Can you work these out from the model? Positions are in its coordinate system, mm. A direction names the side the tool comes from. Coordinates: 2 decimals unless noted, no trailing zeros. Loops run counter-clockwise (first coordinate to the right, second up) from the corner with the lowest first, then second, coordinate; pieces in that order, holes last. Notation, with made-up numbers: (-37, -17.75) - (-2, -17.75) arc R17 cw to (-2, -7.75) - close; hole circle Ø9 at (-40, 40.25). An arc over 180 degrees is marked (long way). Put each result on its own line as item: value. Start each with the question number.
from build123d import *

# Parameters (mm, degrees)
SKETCH1_W               = 8
SKETCH1_H               = 8
BOSS_EXTRUDE1_DEPTH     = 3
CUT_EXTRUDE1_DEPTH      = 12.704699911
CUT_EXTRUDE1_DEPTH_BACK = 12.704699911
CUT_EXTRUDE2_DEPTH      = 11
SKETCH4_R               = 1.75
CUT_EXTRUDE3_DEPTH      = 0.4
SKETCH5_W               = 8
SKETCH5_H               = 1
BOSS_EXTRUDE2_DEPTH     = 2
FILLET1_R               = 4
CUT_EXTRUDE4_DEPTH      = 0.4
CUT_EXTRUDE5_DEPTH      = 0.5


with BuildPart() as part:
    # Sketch1 → Boss-Extrude1 (new body)
    with BuildSketch(Plane(origin=(0, 0, 0), x_dir=(1, 0, 0), z_dir=(0, 1, 0))):
        with Locations((4, 4)):
            Rectangle(SKETCH1_W, SKETCH1_H)
    extrude(amount=BOSS_EXTRUDE1_DEPTH)

    # Sketch2 → Cut-Extrude1 (cut, two sides: drawn at the far end of the back side and taken through both)
    with BuildSketch(Plane.XY.offset(-CUT_EXTRUDE1_DEPTH_BACK)):
        Polygon((0, 0), (0.6, 3), (0, 3), align=None)
        Polygon((8, 0), (7.4, 3), (8, 3), align=None)
    extrude(amount=CUT_EXTRUDE1_DEPTH + CUT_EXTRUDE1_DEPTH_BACK, mode=Mode.SUBTRACT)

    # Sketch3 → Cut-Extrude2 (cut)
    with BuildSketch(Plane(origin=(0, 0, 0), x_dir=(0, 0, -1), z_dir=(1, 0, 0))):
        Polygon((0, 0), (0.6, 3), (0, 3), align=None)
        Polygon((8, 3), (7.4, 3), (8, 0), align=None)
    extrude(amount=CUT_EXTRUDE2_DEPTH, mode=Mode.SUBTRACT)

    # Sketch4 → Cut-Extrude3 (cut)
    with BuildSketch(Plane.XZ):
        with Locations(Location((4, -3.75, 0), (0, 0, 270))):
            Circle(SKETCH4_R)
    extrude(amount=-CUT_EXTRUDE3_DEPTH, mode=Mode.SUBTRACT)

    # Sketch5 → Boss-Extrude2 (add)
    with BuildSketch(Plane.XZ):
        with Locations((4, -7.5)):
            Rectangle(SKETCH5_W, SKETCH5_H)
    extrude(amount=BOSS_EXTRUDE2_DEPTH)

    # Fillet1
    # the kernel refuses this fillet: 4 mm, written as the material it takes off along each edge
    with BuildSketch(Plane(origin=(8, -2, -16.660254038), x_dir=(0, 1, 0), z_dir=(0, 0, 1)), Plane(origin=(0, -2, 1.660254038), x_dir=(0, 1, 0), z_dir=(0, 0, -1))) as fillet1_piece_1:
        with BuildLine():
            CenterArc((4, 3.464101615), FILLET1_R, 180, 60)
            Line((0, 3.464101615), (-0.08, 3.464101615))
            Line((-0.08, 3.464101615), (-0.08, 0))
            Line((-0.08, 0), (0, -0.08))
            ThreePointArc((0, -0.08), (1, -0.08), (1.96, -0.069282032))
            Line((1.96, -0.069282032), (2, 0))
        make_face()
    extrude(amount=18.320508076, mode=Mode.SUBTRACT)

    # Sketch6 → Cut-Extrude4 (cut)
    with BuildSketch(Plane(origin=(0, 3, 0), x_dir=(1, 0, 0), z_dir=(0, 1, 0))):
        with BuildLine():
            Line((2.312898911, 2.041410717), (2.312898911, 6.041410717))
            Line((2.312898911, 6.041410717), (3.991584808, 6.041410717))
            add(Edge.make_bspline(
                [(3.991584808, 6.041410717), (4.042601732, 6.041096301), (4.140920681, 6.040490364), (4.283109063, 6.036071747), (4.414238667, 6.026814487), (4.534891188, 6.016330564), (4.644487122, 6.001077132), (4.74345979, 5.982803671), (4.831642566, 5.961627249), (4.910322089, 5.936265049), (4.982061831, 5.90723713), (5.04889092, 5.87268574), (5.111544162, 5.83220454), (5.170983849, 5.787188805), (5.227461685, 5.737569368), (5.279429347, 5.682033053), (5.32779225, 5.621406813), (5.372511371, 5.556195062), (5.411906117, 5.48668575), (5.447902572, 5.415111184), (5.477205044, 5.340709703), (5.50140862, 5.263831792), (5.52074281, 5.184644366), (5.534162371, 5.102946099), (5.542540058, 5.018884869), (5.543287935, 4.962103945), (5.543668142, 4.93323764)],
                knots=[0, 0, 0, 0, 1.675828044, 3.229627355, 4.67171229, 5.993455049, 7.206927059, 8.304770529, 9.29850117, 10.183580433, 11.017754134, 11.837875825, 12.650738409, 13.464925643, 14.285328857, 15.117007378, 15.959673368, 16.830859064, 17.711229498, 18.58228265, 19.460420693, 20.334473227, 21.228207035, 22.135446768, 23.052097822, 24, 24, 24, 24], degree=3))
            add(Edge.make_bspline(
                [(5.543668142, 4.93323764), (5.542962916, 4.896874176), (5.541584712, 4.825809944), (5.528901745, 4.721651895), (5.5100643, 4.622136315), (5.483211668, 4.527125334), (5.446289845, 4.437736414), (5.403428122, 4.352717347), (5.352308317, 4.272356517), (5.293277733, 4.19745058), (5.226389218, 4.127933229), (5.151349641, 4.065235076), (5.06869476, 4.009111084), (4.977924564, 3.959884897), (4.879671091, 3.917801842), (4.77350828, 3.882394441), (4.659916733, 3.853576761), (4.580902516, 3.840017181), (4.540463013, 3.833077384)],
                knots=[0, 0, 0, 0, 1.05911256, 2.069797862, 3.05271628, 4.008392045, 4.940519534, 5.866323021, 6.779546087, 7.71056835, 8.640711998, 9.585328432, 10.554502533, 11.547017206, 12.589327225, 13.664782803, 14.804835066, 16, 16, 16, 16], degree=3))
            add(Edge.make_bspline(
                [(4.540463013, 3.833077384), (4.579572554, 3.807174767), (4.656115253, 3.756479818), (4.762017587, 3.672984601), (4.857092756, 3.585349912), (4.929078878, 3.507419696), (4.984392794, 3.438888442), (5.028929947, 3.378950347), (5.076970406, 3.309970293), (5.128042999, 3.231910907), (5.183657562, 3.145462828), (5.241745689, 3.049302835), (5.303522957, 2.944368887), (5.345058377, 2.871067212), (5.366584808, 2.833077384)],
                knots=[0, 0, 0, 0, 1.285445069, 2.515791127, 3.691898215, 4.826622834, 5.420063933, 6.105349801, 6.873086501, 7.723915395, 8.66222816, 9.690593598, 10.803111229, 12, 12, 12, 12], degree=3))
            Line((5.366584808, 2.833077384), (5.851360449, 2.041410717))
            Line((5.851360449, 2.041410717), (4.952321988, 2.041410717))
            Line((4.952321988, 2.041410717), (4.383411731, 2.949263281))
            add(Edge.make_bspline(
                [(4.383411731, 2.949263281), (4.357283981, 2.985622121), (4.307400733, 3.055038622), (4.235391184, 3.153681722), (4.169508837, 3.241491798), (4.111507042, 3.319740728), (4.058450932, 3.386209972), (4.011951502, 3.442057857), (3.972955886, 3.488482798), (3.928832249, 3.534515131), (3.877499082, 3.581823547), (3.813952721, 3.627691749), (3.748696505, 3.664257396), (3.678779681, 3.692157844), (3.597922987, 3.71161189), (3.500720436, 3.724006591), (3.384115753, 3.733151261), (3.299833928, 3.733519777), (3.254405321, 3.73371841)],
                knots=[0, 0, 0, 0, 1.465447777, 2.797841088, 3.997266218, 5.05856206, 5.985598736, 6.780315439, 7.437430484, 7.969193402, 8.866571936, 9.718200644, 10.52825214, 11.309096006, 12.174169268, 13.242355782, 14.513606761, 16, 16, 16, 16], degree=3))
            Line((3.254405321, 3.73371841), (3.08212968, 3.73371841))
            Line((3.08212968, 3.73371841), (3.08212968, 2.041410717))
            Line((3.08212968, 2.041410717), (2.312898911, 2.041410717))
        make_face()
        with BuildLine():
            Line((3.08212968, 4.400385076), (3.701520706, 4.400385076))
            add(Edge.make_bspline(
                [(3.701520706, 4.400385076), (3.749332843, 4.400487541), (3.840423044, 4.400682752), (3.969955122, 4.403510317), (4.085670885, 4.405910235), (4.186877859, 4.411940131), (4.274028855, 4.417916326), (4.346774263, 4.425683211), (4.405726987, 4.434863419), (4.464610849, 4.449136231), (4.52492793, 4.474003789), (4.589214527, 4.509422512), (4.644158691, 4.555370201), (4.691753027, 4.608490376), (4.728060837, 4.670937972), (4.756498441, 4.739930879), (4.770916908, 4.817002181), (4.773239296, 4.87042263), (4.774437372, 4.89798123)],
                knots=[0, 0, 0, 0, 1.697953026, 3.23488743, 4.60134403, 5.807846676, 6.835100678, 7.703488618, 8.405232423, 8.952775585, 9.851109663, 10.713519226, 11.549115941, 12.382556273, 13.233359028, 14.101746968, 15.020727134, 16, 16, 16, 16], degree=3))
            add(Edge.make_bspline(
                [(4.774437372, 4.89798123), (4.773074786, 4.928811222), (4.770445895, 4.98829272), (4.749714088, 5.072935459), (4.713527564, 5.147705664), (4.663829732, 5.212726785), (4.601441933, 5.267631557), (4.527131165, 5.311213996), (4.441449505, 5.343672387), (4.379650359, 5.355659208), (4.347354039, 5.361923538)],
                knots=[0, 0, 0, 0, 1.062977961, 2.050844577, 2.982300261, 3.90936959, 4.856017476, 5.831122378, 6.86654153, 8, 8, 8, 8], degree=3))
            add(Edge.make_bspline(
                [(4.347354039, 5.361923538), (4.336678458, 5.363096555), (4.311375089, 5.365876852), (4.266692338, 5.367662514), (4.20955971, 5.370407271), (4.139285669, 5.371528992), (4.056498042, 5.373495271), (3.960867626, 5.373856329), (3.852698247, 5.375009885), (3.776307493, 5.374835906), (3.735975834, 5.374744051)],
                knots=[0, 0, 0, 0, 0.42127143, 0.998501726, 1.753681744, 2.66564073, 3.755712164, 5.002818897, 6.417592707, 8, 8, 8, 8], degree=3))
            Line((3.735975834, 5.374744051), (3.08212968, 5.374744051))
            Line((3.08212968, 5.374744051), (3.08212968, 4.400385076))
        make_face(mode=Mode.SUBTRACT)
    extrude(amount=-CUT_EXTRUDE4_DEPTH, mode=Mode.SUBTRACT)

    # Sketch7 → Cut-Extrude5 (cut)
    with BuildSketch(Plane(origin=(0, 3, 0), x_dir=(1, 0, 0), z_dir=(0, 1, 0))):
        Polygon((6.546707708, 0.907912363), (6.546707708, 1.256630312), (5.871066683, 1.256630312), (5.871066683, 1.53894201), (6.589956907, 2.586117491), (6.873630785, 2.586117491), (6.873630785, 1.539963645), (7.091579503, 1.539963645), (7.091579503, 1.256630312), (6.873630785, 1.256630312), (6.873630785, 0.907912363), align=None)
        Polygon((6.546707708, 1.539963645), (6.546707708, 2.105949222), (6.157805465, 1.539963645), align=None, mode=Mode.SUBTRACT)
    extrude(amount=-CUT_EXTRUDE5_DEPTH, mode=Mode.SUBTRACT)


solid = part.part
Q1. I want a section at B-B on z = -7.5. List the corners of the cut face in (x, y) for me.
Q2. I want a section at A-A on x = 2.75. List the corners of the cut face in (y, z) for me.
Q3. Please list where these lines run through material, in increasing order: line 1 along Y through (x, z) = (1.5, -3.5); line 2 along Z through (x, y) = (3.5, -1.5); line 3 along Y through (x, z) = (3.75, -5). Write a range as [from, to].
Q4. We'd pull the mould along Z, two halves only. Please class faces 1 (the flat face through (3.9, 1.5, -0.3)), 2 (the flat face through (4, 3, -5)), 3 (the flat face through (4, 0.4, -4)): released by +Z, released by -Z, zero draft, split by the parting line, or undercut.
Q5. I want a section at D-D on x = 1. List the corners of the cut face in (y, z) for me.
Q6. On a 3-axis mill with a long thin cutter (end or side, diameter ignored), from which of +Z, -Z, +X, -X, +Y, -Y can I reach the whole of each face in a straight line? I mean faces 4 (the cylindrical face through (2.94, 0.2, -2.36)), 5 (the flat face through (4, 2.6, -4)), 6 (the flat face through (3, 0, -2)). Say none if no direction works.
Q7. I want a section at C-C on y = 1.35. List the corners of the cut face in (x, z) for me.
Q8. Will this pin go through, and if not, where does the flat tip stop? pin 1 (2 mm diameter, centred on x = 5, z = -1, fed in from -Y).
Calculated:
1. outline: (0, 0) arc R4 ccw to (3.46, -2) - (4.54, -2) arc R4 ccw to (8, 0) - (7.5, 2.5) - (0.5, 2.5) - close
2. outline: (-1.94, -8) - (0, -8) - (3, -7.4) - (3, -6.04) - (2.6, -6.04) - (2.6, -2.04) - (3, -2.04) - (3, -0.6) - (0, 0) - (0, -2.53) - (0.4, -2.53) - (0.4, -4.97) - (0, -4.97) - (0, -7) - (-1.94, -7) - close
3. line 1: [0, 3]
3. line 2: [-8, -7]
3. line 3: [0.4, 3]
4. face 1: released by +Z
4. face 2: zero draft
4. face 3: undercut
5. outline: (-1.15, -8) - (0, -8) - (3, -7.4) - (3, -0.6) - (0, 0) - (0, -7) - (-1.15, -7) - close
6. face 4: -Y
6. face 5: +Y
6. face 6: +Z, +X, -X, -Y
7. outline: (0.27, -7.73) - (7.73, -7.73) - (7.73, -0.27) - (0.27, -0.27) - close
8. pin 1: y = 0
